Verification items for the finished model (mm, model axes). A direction names the side the tool comes from. Coordinates: 2 decimals unless noted, no trailing zeros. Write each loop counter-clockwise with the first axis right and the second up, starting at its lowest first coordinate (ties: lowest second). Pieces come first, ordered by that corner, then holes.
```python
from build123d import *

# Parameters (mm, degrees)
CROQUIS1_R              = 3.25
SALIENTE_EXTRUIR1_DEPTH = 35
CORTAR_EXTRUIR1_REACH   = 116.435
CROQUIS2_W              = 8
CROQUIS2_H              = 25
REDONDEO1_R             = 0.5
CROQUIS4_W              = 27
CROQUIS4_H              = 37
CORTAR_EXTRUIR2_DEPTH   = 115.435178158


with BuildPart() as part:
    # Croquis1 → Saliente-Extruir1 (new body)
    with BuildSketch(Plane(origin=(0, 0, 0), x_dir=(0, 0, -1), z_dir=(1, 0, 0))):
        Polygon((0, 10), (0, -10), (10, -10), (10, -5), (13.55, -0.769274746), (17.1, -5), (17.1, -10), (107.1, -10), (107.1, 10), (17.1, 10), (17.1, 5), (10, 5), (10, 10), align=None)
        with Locations((100.1, 0)):
            Circle(CROQUIS1_R, mode=Mode.SUBTRACT)
    extrude(amount=SALIENTE_EXTRUIR1_DEPTH)

    # Croquis2 → Cortar-Extruir1 (cut, up to next)
    with BuildSketch(Plane(origin=(0, 10, 0), x_dir=(1, 0, 0), z_dir=(0, 1, 0)), mode=Mode.PRIVATE) as cortar_extruir1_sk1:
        with Locations((17.5, 94.6)):
            Rectangle(CROQUIS2_W, CROQUIS2_H)
    cortar_extruir1_tool1 = extrude(cortar_extruir1_sk1.sketch, amount=-CORTAR_EXTRUIR1_REACH, mode=Mode.PRIVATE) & part.part
    add(cortar_extruir1_tool1.solids().sort_by_distance((17.5, 10, -94.6))[0], mode=Mode.SUBTRACT)

    # Redondeo1
    redondeo1_edges = [part.edges().sort_by_distance(p)[0] for p in [
        (17.5, -0.769274746, -13.55),
    ]]
    fillet(redondeo1_edges, radius=REDONDEO1_R)

    # Croquis4 → Cortar-Extruir2 (cut, through all)
    with BuildSketch(Plane(origin=(0, 10, 0), x_dir=(1, 0, 0), z_dir=(0, 1, 0))):
        with Locations((17.5, 43.6)):
            Rectangle(CROQUIS4_W, CROQUIS4_H)
    extrude(amount=-CORTAR_EXTRUIR2_DEPTH, mode=Mode.SUBTRACT)


solid = part.part
```
1. Tool access check on faces 1 (the flat face through (17.26, -3.14, -11.56)), 2 (the flat face through (17, 7, -10)), 3 (the flat face through (31, 0, -43)), 4 (the flat face through (13.5, 0, -94)). Record the directions out of +Z, -Z, +X, -X, +Y, -Y that give a thin tool (end or side, any length) a straight path to the whole face; none if there is none.
2. Sectioned sample at C-C, the plane x = 5. Record the boundary of the cut face in (y, z), and give its area (3 significant figures).
3. Draft check along X on faces 5 (the flat face through (0, 0, -53)), 6 (the flat face through (4, 0, -43)), 7 (the flat face through (17, 10, -63)). Enter one of: pulls with the +X half, pulls with the -X half, needs draft (parallel to the pull), parting line crosses it, or undercut.
4. Gauge pin test, flat ends, axial feed: P1, Ø5.5, axis at x = 15.5, y = 8.5, coming from the +Z side; P2, Ø1, axis at x = 3.5, z = -14, coming from the -Y side; P3, Ø12, axis at x = 22.5, z = -43, coming from the -Y side. Record the tip position at first contact, or that the pin passes through.
5. Sectioned sample at B-B, the plane z = -85.5. Record the boundary of the cut face in (x, y).
6. Material ranges on L1, parallel to Z at x = 21, y = 7; L2, parallel to Z at x = 4.75, y = 0; L3, parallel to X at y = -4, z = -44, recorded low to high.
7. Sectioned sample at D-D, the plane y = 0. Record the boundary of the cut face in (x, z), and give its area (3 significant figures).
8. Sectioned sample at A-A, the plane y = -6. Record the boundary of the cut face in (x, z), and give its area (3 significant figures).
Outcome:
1. face 1: +X, -X, -Y
1. face 2: +X, -X, +Y
1. face 3: +Y, -Y
1. face 4: -Z, +Y, -Y
2. outline: (-10, -107.1) - (10, -107.1) - (10, -62.1) - (-10, -62.1) - close; (-10, -25.1) - (10, -25.1) - (10, -17.1) - (5, -17.1) - (5, -10) - (10, -10) - (10, 0) - (-10, 0) - (-10, -10) - (-5, -10) - (-1.23, -13.17) arc R0.5 cw to (-1.23, -13.93) - (-5, -17.1) - (-10, -17.1) - close; hole circle Ø6.5 at (0, -100.1)
2. area: 1,280 mm2
3. face 5: pulls with the -X half
3. face 6: undercut
3. face 7: needs draft
4. P1: stops at z = 0
4. P2: stops at y = -1.9
4. P3: passes through
5. outline: (0, -10) - (13.5, -10) - (13.5, 10) - (0, 10) - close; (21.5, -10) - (35, -10) - (35, 10) - (21.5, 10) - close
6. L1: z = -82.1 to -62.1, -25.1 to -17.1, -10 to 0
6. L2: z = -107.1 to -103.35, -96.85 to -62.1, -25.1 to 0
6. L3: x = 0 to 4, 31 to 35
7. outline: (0, -107.1) - (13.5, -107.1) - (13.5, -103.35) - (0, -103.35) - close; (0, -96.85) - (13.5, -96.85) - (13.5, -82.1) - (21.5, -82.1) - (21.5, -96.85) - (35, -96.85) - (35, 0) - (0, 0) - close; (21.5, -107.1) - (35, -107.1) - (35, -103.35) - (21.5, -103.35) - close; hole (4, -62.1) - (31, -62.1) - (31, -25.1) - (4, -25.1) - close
7. area: 2,370 mm2
8. outline: (0, -107.1) - (13.5, -107.1) - (13.5, -82.1) - (21.5, -82.1) - (21.5, -107.1) - (35, -107.1) - (35, -17.1) - (0, -17.1) - close; (0, -10) - (35, -10) - (35, 0) - (0, 0) - close; hole (4, -62.1) - (31, -62.1) - (31, -25.1) - (4, -25.1) - close
8. area: 2,300 mm2
